```python
from build123d import *

# Parameters (mm, degrees)
ESBO_O1_R                = 9
RESSALTO_EXTRUS_O1_DEPTH = 6
FILETE1_R                = 1
CASCA1_T                 = -2
ESBO_O2_W                = 8.35
ESBO_O2_H                = 8.35
ESBO_O2_W_2              = 4.35
ESBO_O2_H_2              = 4.35
RESSALTO_EXTRUS_O2_DEPTH = 4
FILETE2_R                = 1
CORTE_EXTRUS_O2_DEPTH    = 1
ESBO_O6_R                = 11
ESBO_O6_R_2              = 9
RESSALTO_EXTRUS_O3_DEPTH = 0.5
CORTE_EXTRUS_O4_DEPTH    = 17.673332001
ESBO_O8_W                = 4.35
ESBO_O8_H                = 4.35
RESSALTO_EXTRUS_O4_DEPTH = 2


with BuildPart() as part:
    # Esboço1 → Ressalto-extrusão1 (new body)
    with BuildSketch(Plane.XY):
        Circle(ESBO_O1_R)
    extrude(amount=RESSALTO_EXTRUS_O1_DEPTH)

    # Filete1
    filete1_edges = [part.edges().sort_by_distance(p)[0] for p in [
        (-9, 0, 6),
    ]]
    fillet(filete1_edges, radius=FILETE1_R)

    # Casca1
    casca1_openings = [part.faces().sort_by_distance(p)[0] for p in [
        (0, 0, 0),
    ]]
    offset(amount=CASCA1_T, openings=casca1_openings, kind=Kind.INTERSECTION)

    # Esboço2 → Ressalto-extrusão2 (add)
    with BuildSketch(Plane(origin=(0, 0, 4), x_dir=(-1, 0, 0), z_dir=(0, 0, -1))):
        Rectangle(ESBO_O2_W, ESBO_O2_H)
        Rectangle(ESBO_O2_W_2, ESBO_O2_H_2, mode=Mode.SUBTRACT)
    extrude(amount=RESSALTO_EXTRUS_O2_DEPTH)

    # Filete2
    filete2_edges = [part.edges().sort_by_distance(p)[0] for p in [
        (-4.175, -4.175, 2),
        (-4.175, 4.175, 2),
        (4.175, 4.175, 2),
        (4.175, -4.175, 2),
    ]]
    fillet(filete2_edges, radius=FILETE2_R)

    # Esboço4 → Corte-extrusão2 (cut)
    # profile 1 of 8: a face of its own
    with BuildSketch(Plane.XY.offset(6)):
        with BuildLine():
            Line((-0.625, 6.5), (-0.625, 5.3))
            ThreePointArc((-0.625, 5.3), (0, 4.675), (0.625, 5.3))
            Line((0.625, 5.3), (0.625, 6.5))
            ThreePointArc((0.625, 6.5), (0, 7.125), (-0.625, 6.5))
        make_face()
    # profile 2 of 8: a face of its own
    with BuildSketch(Plane.XY.offset(6)):
        with BuildLine():
            Line((-1.5, -4.5), (-1.5, -5.95))
            ThreePointArc((-1.5, -5.95), (-1.280330086, -6.480330086), (-0.75, -6.7))
            Line((-0.75, -6.7), (0.75, -6.7))
            ThreePointArc((0.75, -6.7), (1.280330086, -6.480330086), (1.5, -5.95))
            Line((1.5, -5.95), (1.5, -4.5))
            ThreePointArc((1.5, -4.5), (2.102155122, -3.101716024), (3.036856928, -1.9))
            ThreePointArc((3.036856928, -1.9), (0, 4.05), (-3.036856928, -1.9))
            ThreePointArc((-3.036856928, -1.9), (-2.102155122, -3.101716024), (-1.5, -4.5))
        make_face()
        with BuildLine():
            Line((-0.842764128, -4.084062043), (0.842764128, -4.084062043))
            ThreePointArc((0.842764128, -4.084062043), (1.495755637, -2.654539881), (2.461620284, -1.414766916))
            ThreePointArc((2.461620284, -1.414766916), (0, 3.3), (-2.461620284, -1.414766916))
            ThreePointArc((-2.461620284, -1.414766916), (-1.495755637, -2.654539881), (-0.842764128, -4.084062043))
        make_face(mode=Mode.SUBTRACT)
        with BuildLine():
            Line((-0.75, -4.834062043), (0.75, -4.834062043))
            Line((0.75, -4.834062043), (0.75, -5.7))
            ThreePointArc((0.75, -5.7), (0.676776695, -5.876776695), (0.5, -5.95))
            Line((0.5, -5.95), (-0.5, -5.95))
            ThreePointArc((-0.5, -5.95), (-0.676776695, -5.876776695), (-0.75, -5.7))
            Line((-0.75, -5.7), (-0.75, -4.834062043))
        make_face(mode=Mode.SUBTRACT)
    # profile 3 of 8: a face of its own
    with BuildSketch(Plane.XY.offset(6)):
        with BuildLine():
            Line((3.942120305, 5.126003782), (3.093592168, 4.277475644))
            ThreePointArc((3.093592168, 4.277475644), (3.093592168, 3.393592168), (3.977475644, 3.393592168))
            Line((3.977475644, 3.393592168), (4.826003782, 4.242120305))
            ThreePointArc((4.826003782, 4.242120305), (4.826003782, 5.126003782), (3.942120305, 5.126003782))
        make_face()
    # profile 4 of 8: a face of its own
    with BuildSketch(Plane.XY.offset(6)):
        with BuildLine():
            Line((6.2, 0.925), (5, 0.925))
            ThreePointArc((5, 0.925), (4.375, 0.3), (5, -0.325))
            Line((5, -0.325), (6.2, -0.325))
            ThreePointArc((6.2, -0.325), (6.825, 0.3), (6.2, 0.925))
        make_face()
    # profile 5 of 8: a face of its own
    with BuildSketch(Plane.XY.offset(6)):
        with BuildLine():
            Line((4.826003782, -3.642120305), (3.977475644, -2.793592168))
            ThreePointArc((3.977475644, -2.793592168), (3.093592168, -2.793592168), (3.093592168, -3.677475644))
            Line((3.093592168, -3.677475644), (3.942120305, -4.526003782))
            ThreePointArc((3.942120305, -4.526003782), (4.826003782, -4.526003782), (4.826003782, -3.642120305))
        make_face()
    # profile 6 of 8: a face of its own
    with BuildSketch(Plane.XY.offset(6)):
        with BuildLine():
            Line((-3.942120305, -4.526003782), (-3.093592168, -3.677475644))
            ThreePointArc((-3.093592168, -3.677475644), (-3.093592168, -2.793592168), (-3.977475644, -2.793592168))
            Line((-3.977475644, -2.793592168), (-4.826003782, -3.642120305))
            ThreePointArc((-4.826003782, -3.642120305), (-4.826003782, -4.526003782), (-3.942120305, -4.526003782))
        make_face()
    # profile 7 of 8: a face of its own
    with BuildSketch(Plane.XY.offset(6)):
        with BuildLine():
            Line((-6.2, -0.325), (-5, -0.325))
            ThreePointArc((-5, -0.325), (-4.375, 0.3), (-5, 0.925))
            Line((-5, 0.925), (-6.2, 0.925))
            ThreePointArc((-6.2, 0.925), (-6.825, 0.3), (-6.2, -0.325))
        make_face()
    # profile 8 of 8: a face of its own
    with BuildSketch(Plane.XY.offset(6)):
        with BuildLine():
            Line((-4.826003782, 4.242120305), (-3.977475644, 3.393592168))
            ThreePointArc((-3.977475644, 3.393592168), (-3.093592168, 3.393592168), (-3.093592168, 4.277475644))
            Line((-3.093592168, 4.277475644), (-3.942120305, 5.126003782))
            ThreePointArc((-3.942120305, 5.126003782), (-4.826003782, 5.126003782), (-4.826003782, 4.242120305))
        make_face()
    extrude(amount=-CORTE_EXTRUS_O2_DEPTH, mode=Mode.SUBTRACT)

    # Esboço6 → Ressalto-extrusão3 (add)
    with BuildSketch(Plane(origin=(0, 0, 0), x_dir=(-1, 0, 0), z_dir=(0, 0, -1))):
        Circle(ESBO_O6_R)
        Circle(ESBO_O6_R_2, mode=Mode.SUBTRACT)
    extrude(amount=-RESSALTO_EXTRUS_O3_DEPTH)

    # Esboço7 → Corte-extrusão4 (cut, through all)
    with BuildSketch(Plane(origin=(0, 0, 0), x_dir=(-1, 0, 0), z_dir=(0, 0, -1))):
        with BuildLine():
            Line((-10, 4.582575695), (-10, -4.582575695))
            ThreePointArc((-10, -4.582575695), (-11, 0), (-10, 4.582575695))
        make_face()
        with BuildLine():
            Line((10, 4.582575695), (10, -4.582575695))
            ThreePointArc((10, -4.582575695), (11, 0), (10, 4.582575695))
        make_face()
    extrude(amount=-CORTE_EXTRUS_O4_DEPTH, mode=Mode.SUBTRACT)

    # Esboço8 → Ressalto-extrusão4 (add)
    with BuildSketch(Plane(origin=(0, 0, 4), x_dir=(-1, 0, 0), z_dir=(0, 0, -1))):
        Rectangle(ESBO_O8_W, ESBO_O8_H)
    extrude(amount=RESSALTO_EXTRUS_O4_DEPTH)


solid = part.part
```
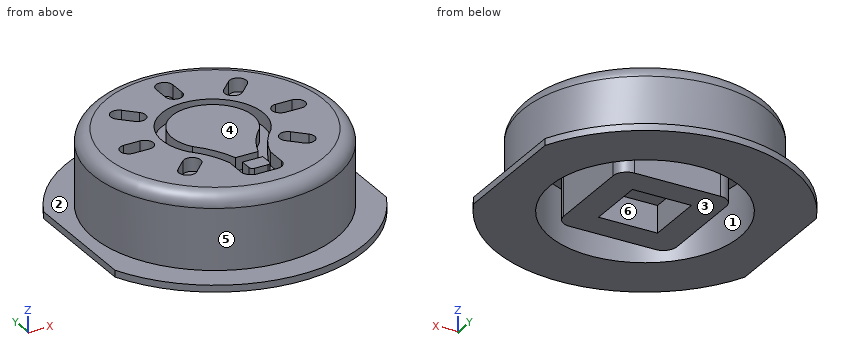
Part model, mm, in its own coordinate system. Face numbers are marked on the shaded views. A direction names the side the tool comes from. Coordinates: 2 decimals unless noted, no trailing zeros. Write each loop counter-clockwise with the first axis right and the second up, starting at its lowest first coordinate (ties: lowest second). Pieces come first, ordered by that corner, then holes.
Item 1: Mould opens along Y. For the marked faces 4, 5 and 6 say: released by +Y, released by -Y, zero draft, split by the parting line, or undercut.
Item 2: Slice it at A-A (z = 3.65). Write the cut outline in (x, y) (3 decimals).
Item 3: Which spindle directions (+Z, -Z, +X, -X, +Y, -Y) get a long thin tool onto all of the face, cutting with end or side? Do the marked faces 1, 2 and 3. Say none if no direction does.
Item 4: Probe line 1 (X direction, y = 0, z = 1) (3 decimals); line 2 (X direction, y = 0, z = 2.6) (3 decimals). List the from-to ranges inside material, lowest first.
Item 5: Pin check, flat tips, straight feed: pin 1 (2 mm diameter, centred on y = -0.5, z = 1, fed in from +X); pin 2 (0.8 mm diameter, centred on x = 5.5, z = 5.5, fed in from -Y); pin 3 (1 mm diameter, centred on y = -5.5, z = 5.5, fed in from -X); pin 4 (0.8 mm diameter, centred on y = 6, z = 5.5, fed in from +X). Stop position of each tip, or through.
Results found:
1. face 4: zero draft
1. face 5: split by the parting line
1. face 6: undercut
2. outline: circle Ø18 at (0, 0); (-4.175, -3.175) arc R1 ccw to (-3.175, -4.175) - (3.175, -4.175) arc R1 ccw to (4.175, -3.175) - (4.175, 3.175) arc R1 ccw to (3.175, 4.175) - (-3.175, 4.175) arc R1 ccw to (-4.175, 3.175) - close; hole circle Ø14 at (0, 0)
3. face 1: -Z
3. face 2: +Z
3. face 3: -Z, +X, -X, +Y, -Y
4. line 1: x = -9 to -7, -4.175 to -2.175, 2.175 to 4.175, 7 to 9
4. line 2: x = -9 to -7, -4.175 to 4.175, 7 to 9
5. pin 1: stops at x = 10
5. pin 2: stops at y = -7.32
5. pin 3: stops at x = -7.4
5. pin 4: stops at x = 6.94
